Model file for the job. Use its own axes, mm. Face numbers are marked on the shaded views. A direction names the side the tool comes from. Give positions to 0.01 mm unless a question says otherwise; leave off trailing zeros. Loops run counter-clockwise (first coordinate to the right, second up) from the corner with the lowest first, then second, coordinate; pieces in that order, holes last. Notation, with made-up numbers: (4.25, 59) - (53.25, 59) arc R31 cw to (53.25, 87) - close; hole circle Ø1 at (11, 68.25). An arc over 180 degrees is marked (long way). Use a Markdown table: item, result.
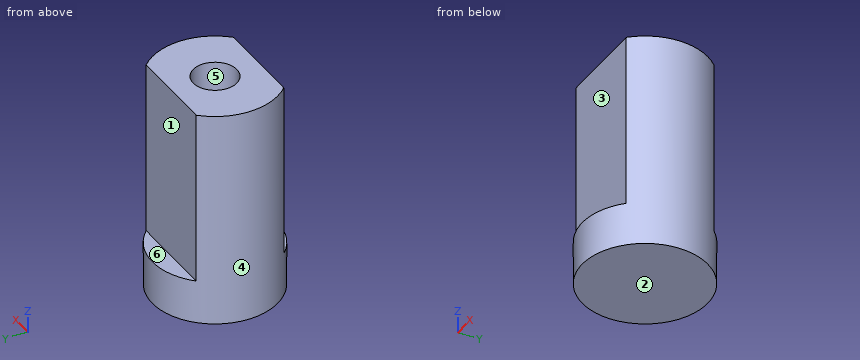
Autodesk Inventor part; units mm, degrees
ref_plane "YZ Plane" through (0, 0, 0) normal (1, 0, 0) x (0, 1, 0)
ref_plane "XZ Plane" through (0, 0, 0) normal (0, 1, 0) x (-1, 0, 0)
ref_plane "XY Plane" through (0, 0, 0) normal (0, 0, 1) x (1, 0, 0)
sketch "Sketch1" plane through (0, 0, 0) normal (0, 0, 1) x (1, 0, 0)
  circle A0 centre (0, 0) radius 2.7305
  dimension "d0" = 5.461
extrude "Extrusion1" add sketch "Sketch1" along normal blind 1.905
sketch "Sketch2" plane through (0, 0, 1.905) normal (0, 0, 1) x (1, 0, 0)
  circle A0 centre (0, 0) radius 2.7305
  line L0 (-1.9562, 1.905) -> (1.9562, 1.905)
  line L1 (1.9562, -1.905) -> (-1.9562, -1.905)
  arc A1 (-1.9562, 1.905) -> (-1.9562, -1.905) centre (0, 0) ccw
  arc A2 (1.9562, -1.905) -> (1.9562, 1.905) centre (0, 0) ccw
  point P0 (0, 1.905)
  point P1 (0, -1.905)
  dimension "d3" = 1.905
  dimension "d4" = 1.905
extrude "Extrusion2" add sketch "Sketch2" along normal blind 7.62 contours A0 L1 L0
sketch "Sketch3" plane through (0, 0, 9.525) normal (0, 0, 1) x (1, 0, 0)
  circle A0 centre (0, 0) radius 2.7305
  circle A1 centre (0, 0) radius 0.9525
  dimension "d7" = 1.905
extrude "Extrusion3" cut sketch "Sketch3" against normal blind 7.62 contours A1
properties part number "MotorShaft" material "ABS Plastic"
(1) Drill centre lines: probe 1 along Y at (x, z) = (0, 8.25) (1 decimal); probe 2 along Z at (x, y) = (0.6, 0.1) (3 decimals); probe 3 along X at (y, z) = (0.45, 6). Where is each one in solid material? Low to high. Write a range as [from, to].
Computed:
| item | result |
|---|---|
| probe 1 | [-1.9, -1], [1, 1.9] |
| probe 2 | [0, 1.905] |
| probe 3 | [-2.69, -0.84], [0.84, 2.69] |
(2) Slice it at C-C, the plane z = 5.75. Write the cut outline in (x, y) (1 decimal), plus the area to 3 significant figures.
Computed:
| item | result |
|---|---|
| outline | (-2, -1.9) - (2, -1.9) arc R2.7 ccw to (2, 1.9) - (-2, 1.9) arc R2.7 ccw to start; hole circle Ø1.9 at (0, 0) |
| area | 16.1 mm² |
(3) Pin check, flat tips, straight feed: P1, Ø1, axis at x = 1, z = 2.5, coming from the -Y side (3 decimals); P2, Ø1.1, axis at x = 0, y = 0, coming from the +Z side (3 decimals); P3, Ø3, axis at x = -1.5, z = 6, coming from the +Y side (3 decimals). Stop position of each tip, or through.
Computed:
| item | result |
|---|---|
| P1 | y = -1.905 |
| P2 | z = 1.905 |
| P3 | y = 1.905 |
(4) Slice it at A-A, the plane x = 0. Write the cut outline in (y, z) (1 decimal), plus the area to 3 significant figures.
Computed:
| item | result |
|---|---|
| outline | (-2.7, 0) - (2.7, 0) - (2.7, 1.9) - (1.9, 1.9) - (1.9, 9.5) - (1, 9.5) - (1, 1.9) - (-1, 1.9) - (-1, 9.5) - (-1.9, 9.5) - (-1.9, 1.9) - (-2.7, 1.9) - close |
| area | 24.9 mm² |
(5) 3-axis set-ups, long thin cutter, end or side, ignore diameter. For the marked faces 1, 2 and 3: which of +Z, -Z, +X, -X, +Y, -Y reach the whole face in a straight line?
Computed:
| item | result |
|---|---|
| face 1 | +Z, +X, -X, +Y |
| face 2 | -Z, +X, -X, +Y, -Y |
| face 3 | +Z, +X, -X, -Y |
(6) Mould opens along X. For the marked faces 4, 5 and 6 say: pulls with the +X half, pulls with the -X half, needs draft (parallel to the pull), parting line crosses it, or undercut.
Computed:
| item | result |
|---|---|
| face 4 | parting line crosses it |
| face 5 | undercut |
| face 6 | needs draft |
(7) Slice it at D-D, the plane z = 1. Write the cut outline in (x, y), plus the area to 3 significant figures.
Computed:
| item | result |
|---|---|
| outline | circle Ø5.46 at (0, 0) |
| area | 23.4 mm² |
(8) Slice it at B-B, the plane y = 0. Write the cut outline in (x, z) (1 decimal).
Computed:
| item | result |
|---|---|
| outline | (-2.7, 0) - (2.7, 0) - (2.7, 9.5) - (1, 9.5) - (1, 1.9) - (-1, 1.9) - (-1, 9.5) - (-2.7, 9.5) - close |
